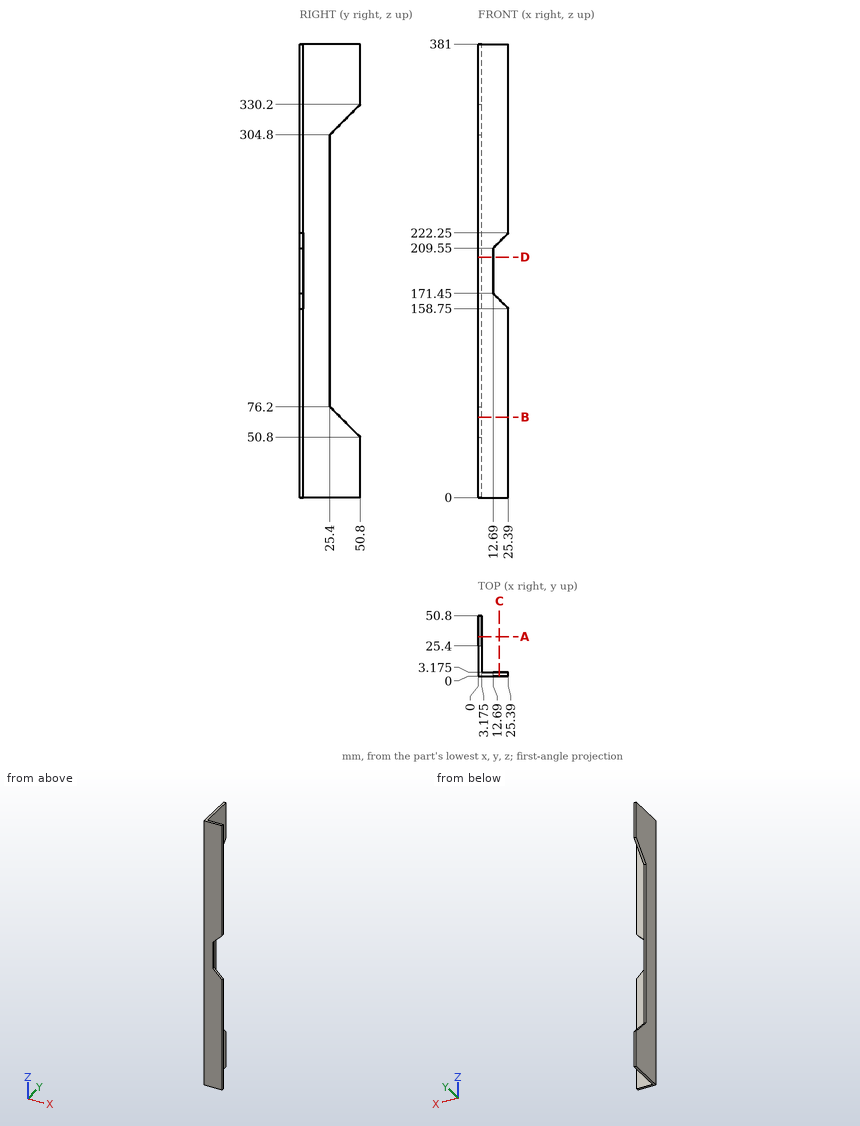
Geometry check sheet. Reference: drawing and pictorial views, mm from the part's lowest x, y, z. Give positions to 0.01 mm unless a question says otherwise; leave off trailing zeros. Order: outer loops, then holes, each group sorted by start corner. A loop starts at its lowest first (then second) coordinate and runs counter-clockwise, first axis right, second up. Notation, with made-up numbers: M 87.5,57 L 125.5,57 A17 ccw 125.5,71 Z; hole C -31,52.25 d3. An arc over 180 degrees is marked long. Answer in a Markdown table with one row per item. Add a question column.
Item 1: Gauge pin test, flat ends, axial feed: pin 1 (1 mm diameter, centred on y = 2, z = 181.5, fed in from +X); pin 2 (4 mm diameter, centred on x = 10.5, z = 194.5, fed in from +Y) (3 decimals); pin 3 (14.5 mm diameter, centred on y = 20.5, z = 193, fed in from +X) (3 decimals). Record the tip position at first contact, or that the pin passes through.
Item 2: Section check B-B, the plane z = 67.5. Enter the section's corners in (x, y) (1 decimal), and give its area (3 significant figures).
Item 3: Section check D-D, the plane z = 202. Enter the section's corners in (x, y) (1 decimal), and give its area (3 significant figures).
Item 4: Section check C-C, the plane x = 17.75. Enter the section's corners in (y, z) (1 decimal).
Item 5: Scan lines: probe 1 along Y at (x, z) = (3, 171); probe 2 along X at (y, z) = (35, 335.5) (3 decimals). Record each from-to range of solid material in increasing order. Write a range as from..to.
Item 6: Section check A-A, the plane y = 33. Enter the section's corners in (x, z) (3 decimals).
Filled sheet:
| question | item | result |
|---|---|---|
| 1 | pin 1 | stops at x = 12.69 |
| 1 | pin 2 | stops at y = 3.175 |
| 1 | pin 3 | stops at x = 3.175 |
| 2 | outline | M 0,0 L 25.4,0 L 25.4,3.2 L 3.2,3.2 L 3.2,34.1 L 0,34.1 Z |
| 2 | area | 179 mm^2 |
| 3 | outline | M 0,0 L 12.7,0 L 12.7,3.2 L 3.2,3.2 L 3.2,25.4 L 0,25.4 Z |
| 3 | area | 111 mm^2 |
| 4 | outline | M 0,0 L 3.2,0 L 3.2,166.4 L 0,166.4 Z; M 0,214.6 L 3.2,214.6 L 3.2,381 L 0,381 Z |
| 5 | probe 1 | y = 0..25.4 |
| 5 | probe 2 | x = 0..3.175 |
| 6 | outline | M 0,0 L 3.175,0 L 3.175,68.6 L 0,68.6 Z; M 0,312.4 L 3.175,312.4 L 3.175,381 L 0,381 Z |
